Here's how the part is built. I have some questions about the finished solid (model axes, mm). A direction names the side the tool comes from. Round coordinates to 2 decimals unless told otherwise and drop trailing zeros. Write each loop counter-clockwise with the first axis right and the second up, starting at its lowest first coordinate (ties: lowest second). Pieces come first, ordered by that corner, then holes. Notation, with made-up numbers: (50, 74) - (81, 74) arc R27 ccw to (81, 113) - close; hole circle Ø7 at (8.25, 16). An arc over 180 degrees is marked (long way). Use one line per item in the form item = value. Start each with the question number.
1. Which directions (+Z, -Z, +X, -X, +Y, -Y) give clear straight access to the entire face, cutting with the end or side of a thin tool? Please do faces 3 (the flat face through (2.3, 2.45, 1.01)), 4 (the flat face through (-7.965, -0.075, 1.014)).
2. We'd pull the mould along Y, two halves only. Please class faces 1 (the cylindrical face through (11.923, 3.755, 2.958)), 2 (the flat face through (4.767, -1.197, 1.014)): +Y half, -Y half, draft (parallel to the pull), parting line (faces both ways), or undercut.
3. If I drill on line 1 along Y through (x, z) = (0, 2.15); line 2 along X through (y, z) = (-0.5, 5.15); line 3 along Y through (x, z) = (6.75, 0.3), over which ranges is the centre line in solid material (lowest first)?
4. Will these pins go through, and if not, where does the flat tip stop? pin 1 (1.5 mm diameter, centred on y = 2, z = 4.5, fed in from -X); pin 2 (1 mm diameter, centred on y = 9, z = 4.5, fed in from +X); pin 3 (1.5 mm diameter, centred on y = -6, z = 3.5, fed in from -X).
5. I want a section at B-B, the plane z = 1.1. State how many separate pieces and enclosed holes the cut face has, plus the area to 3 significant figures.
6. I want a section at A-A, the plane z = 3. List the corners of the cut face in (x, y) for me.
```python
from build123d import *

# Parameters (mm, degrees)
F0_R     = 12.5
F1_DEPTH = 6
F2_R     = 10
F2_R_2   = 3
F3_DEPTH = 4
F5_D     = 3.5
F7_DEPTH = 25
F8_DEPTH = 25
F9_DEPTH = 25


with BuildPart() as f1:
    # F0 (on Top) → F1 (new body)
    with BuildSketch(Plane.XY):
        Circle(F0_R)
    extrude(amount=F1_DEPTH)

    # F2 (on face) → F3 (cut)
    with BuildSketch(Plane.XY.offset(6)):
        Circle(F2_R)
        Circle(F2_R_2, mode=Mode.SUBTRACT)
    extrude(amount=-F3_DEPTH, mode=Mode.SUBTRACT)

    # F5 (through all)
    with Locations(Plane.XY.offset(6)):
        with Locations((0, 0)):
            Hole(F5_D / 2)

    # F6 (on face) → F7 (cut)
    with BuildSketch(Plane.XY.offset(2)):
        Polygon((-6.076968, 0.687006), (-6.376841, 2.190097), (-7.828492, 2.681945), (-8.980271, 1.670702), (-8.680398, 0.167611), (-7.228746, -0.324237), align=None)
        Polygon((-3.746789, -7.621035), (-2.120291, -5.845455), (-2.844739, -3.549077), (-5.195685, -3.028278), (-6.822183, -4.803858), (-6.097735, -7.100236), align=None)
        Polygon((-4.772137, 3.967759), (-3.990072, 5.552483), (-4.971451, 7.022133), (-6.734895, 6.907059), (-7.516959, 5.322335), (-6.53558, 3.852685), align=None)
        Polygon((-0.476487, 4.366405), (0.474315, 5.646003), (-0.158448, 7.109221), (-1.742013, 7.292841), (-2.692815, 6.013243), (-2.060052, 4.550025), align=None)
        Polygon((1.836744, 5.509974), (3.602874, 5.897518), (4.150317, 7.620804), (2.931629, 8.956546), (1.165498, 8.569002), (0.618056, 6.845716), align=None)
        Polygon((3.627879, 0.757783), (5.067878, 1.502148), (5.143239, 3.121406), (3.778601, 3.9963), (2.338601, 3.251935), (2.26324, 1.632677), align=None)
        Polygon((4.707175, -4.991184), (4.856818, -3.136321), (3.325281, -2.079295), (1.6441, -2.877132), (1.494457, -4.731995), (3.025994, -5.789022), align=None)
        Polygon((7.328884, -1.39316), (7.034425, 0), (5.680684, 0.441571), (4.621402, -0.510017), (4.91586, -1.903177), (6.269601, -2.344748), align=None)
        Polygon((-4.28992, -1.446621), (-3.774462, -0.835584), (-4.045906, -0.083666), (-4.832809, 0.057215), (-5.348267, -0.553822), (-5.076822, -1.30574), align=None)
        Polygon((0.89645, -8.866839), (1.712371, -7.360636), (0.815921, -5.900926), (-0.89645, -5.947419), (-1.712371, -7.453623), (-0.815921, -8.913333), align=None)
        Polygon((6.360979, 3.235691), (7.459494, 2.838528), (8.352706, 3.591288), (8.147402, 4.741212), (7.048886, 5.138376), (6.155675, 4.385615), align=None)
    extrude(amount=-F7_DEPTH, mode=Mode.SUBTRACT)

    # F6 (on face) → F8 (cut)
    with BuildSketch(Plane.XY.offset(2)):
        Polygon((-6.076968, 0.687006), (-6.376841, 2.190097), (-7.828492, 2.681945), (-8.980271, 1.670702), (-8.680398, 0.167611), (-7.228746, -0.324237), align=None)
        Polygon((-3.746789, -7.621035), (-2.120291, -5.845455), (-2.844739, -3.549077), (-5.195685, -3.028278), (-6.822183, -4.803858), (-6.097735, -7.100236), align=None)
        Polygon((-4.772137, 3.967759), (-3.990072, 5.552483), (-4.971451, 7.022133), (-6.734895, 6.907059), (-7.516959, 5.322335), (-6.53558, 3.852685), align=None)
        Polygon((-0.476487, 4.366405), (0.474315, 5.646003), (-0.158448, 7.109221), (-1.742013, 7.292841), (-2.692815, 6.013243), (-2.060052, 4.550025), align=None)
        Polygon((1.836744, 5.509974), (3.602874, 5.897518), (4.150317, 7.620804), (2.931629, 8.956546), (1.165498, 8.569002), (0.618056, 6.845716), align=None)
        Polygon((3.627879, 0.757783), (5.067878, 1.502148), (5.143239, 3.121406), (3.778601, 3.9963), (2.338601, 3.251935), (2.26324, 1.632677), align=None)
        Polygon((4.707175, -4.991184), (4.856818, -3.136321), (3.325281, -2.079295), (1.6441, -2.877132), (1.494457, -4.731995), (3.025994, -5.789022), align=None)
        Polygon((7.328884, -1.39316), (7.034425, 0), (5.680684, 0.441571), (4.621402, -0.510017), (4.91586, -1.903177), (6.269601, -2.344748), align=None)
        Polygon((-4.28992, -1.446621), (-3.774462, -0.835584), (-4.045906, -0.083666), (-4.832809, 0.057215), (-5.348267, -0.553822), (-5.076822, -1.30574), align=None)
        Polygon((0.89645, -8.866839), (1.712371, -7.360636), (0.815921, -5.900926), (-0.89645, -5.947419), (-1.712371, -7.453623), (-0.815921, -8.913333), align=None)
        Polygon((6.360979, 3.235691), (7.459494, 2.838528), (8.352706, 3.591288), (8.147402, 4.741212), (7.048886, 5.138376), (6.155675, 4.385615), align=None)
    extrude(amount=-F8_DEPTH, mode=Mode.SUBTRACT)

    # F6 (on face) → F9 (cut)
    with BuildSketch(Plane.XY.offset(2)):
        Polygon((-6.076968, 0.687006), (-6.376841, 2.190097), (-7.828492, 2.681945), (-8.980271, 1.670702), (-8.680398, 0.167611), (-7.228746, -0.324237), align=None)
        Polygon((-3.746789, -7.621035), (-2.120291, -5.845455), (-2.844739, -3.549077), (-5.195685, -3.028278), (-6.822183, -4.803858), (-6.097735, -7.100236), align=None)
        Polygon((-4.772137, 3.967759), (-3.990072, 5.552483), (-4.971451, 7.022133), (-6.734895, 6.907059), (-7.516959, 5.322335), (-6.53558, 3.852685), align=None)
        Polygon((-0.476487, 4.366405), (0.474315, 5.646003), (-0.158448, 7.109221), (-1.742013, 7.292841), (-2.692815, 6.013243), (-2.060052, 4.550025), align=None)
        Polygon((1.836744, 5.509974), (3.602874, 5.897518), (4.150317, 7.620804), (2.931629, 8.956546), (1.165498, 8.569002), (0.618056, 6.845716), align=None)
        Polygon((3.627879, 0.757783), (5.067878, 1.502148), (5.143239, 3.121406), (3.778601, 3.9963), (2.338601, 3.251935), (2.26324, 1.632677), align=None)
        Polygon((4.707175, -4.991184), (4.856818, -3.136321), (3.325281, -2.079295), (1.6441, -2.877132), (1.494457, -4.731995), (3.025994, -5.789022), align=None)
        Polygon((7.328884, -1.39316), (7.034425, 0), (5.680684, 0.441571), (4.621402, -0.510017), (4.91586, -1.903177), (6.269601, -2.344748), align=None)
        Polygon((-4.28992, -1.446621), (-3.774462, -0.835584), (-4.045906, -0.083666), (-4.832809, 0.057215), (-5.348267, -0.553822), (-5.076822, -1.30574), align=None)
        Polygon((0.89645, -8.866839), (1.712371, -7.360636), (0.815921, -5.900926), (-0.89645, -5.947419), (-1.712371, -7.453623), (-0.815921, -8.913333), align=None)
        Polygon((6.360979, 3.235691), (7.459494, 2.838528), (8.352706, 3.591288), (8.147402, 4.741212), (7.048886, 5.138376), (6.155675, 4.385615), align=None)
    extrude(amount=-F9_DEPTH, mode=Mode.SUBTRACT)


solid = f1.part
```
Model answer:
q1.face_3 = -Z
q1.face_4 = +Z, -Z
q2.face_1 = parting line
q2.face_2 = undercut
q3.line_1 = -12.5 to -10, -3 to -1.75, 1.75 to 3, 10 to 12.5
q3.line_2 = -12.49 to -9.99, -2.96 to -1.68, 1.68 to 2.96, 9.99 to 12.49
q3.line_3 = -10.52 to -1.91, 0.09 to 3.1, 4.89 to 10.52
q4.pin_1 = -12.44
q4.pin_2 = 9.17
q4.pin_3 = -11.34
q5.separate_pieces = 1
q5.enclosed_holes = 12
q5.area = 403 mm2
q6.outline = circle Ø25 at (0, 0); circle Ø6 at (0, 0); hole circle Ø20 at (0, 0); hole circle Ø3.5 at (0, 0)
